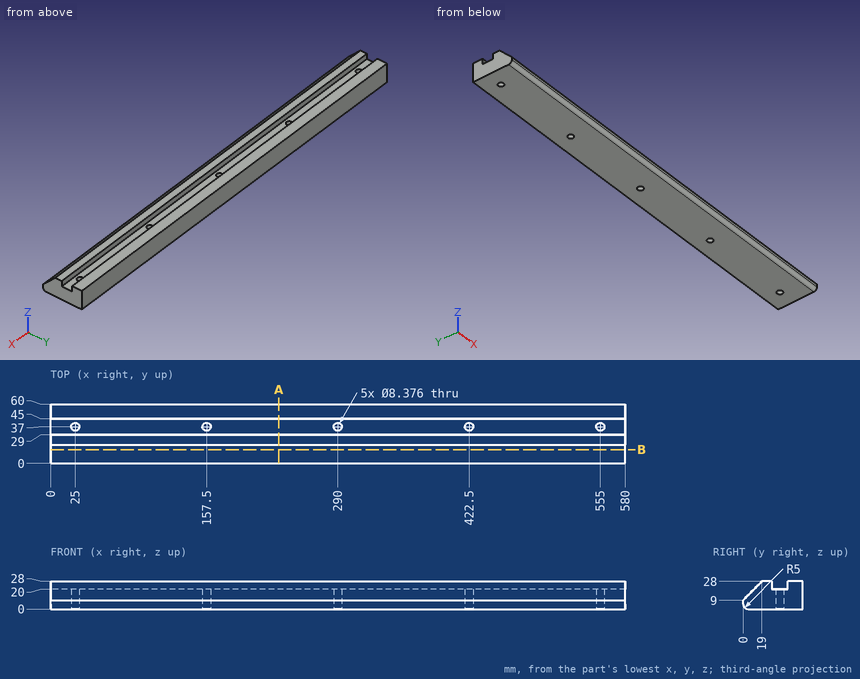
Input: dimensioned drawing with shaded views. Units: mm. Origin: part minimum x, y, z. Give positions to 0.01 mm unless a question says otherwise; leave off trailing zeros. Write each loop counter-clockwise with the first axis right and the second up, starting at its lowest first coordinate (ties: lowest second). Pieces come first, ordered by that corner, then holes.
1. Section query B-B (y = 14). Return the cut outline in (x, z).
2. First-contact query: pin 1 (9 mm diameter, centred on x = 200.5, z = 22, fed in from -Y); pin 2 (3 mm diameter, centred on x = 138.5, y = 35.5, fed in from +Z); pin 3 (10 mm diameter, centred on x = 162.5, z = 19, fed in from -Y). Flat tips, straight axial feed; report the tip coordinate or a pass-through.
3. Material intervals for line 1 along X through (y, z) = (37, 14.25); line 2 along X through (y, z) = (36, 17.5); line 3 along Y through (x, z) = (422.5, 8.25), sorted ascending.
4. Section query A-A (x = 230.5). Return the cut outline in (y, z), then the cut area to 3 significant figures.
Output values:
1. outline: (0, 0) - (580, 0) - (580, 23) - (0, 23) - close
2. pin 1: stops at y = 8.5
2. pin 2: stops at z = 20
2. pin 3: stops at y = 5
3. line 1: x = 0 to 20.81, 29.19 to 153.31, 161.69 to 285.81, 294.19 to 418.31, 426.69 to 550.81, 559.19 to 580
3. line 2: x = 0 to 20.93, 29.07 to 153.43, 161.57 to 285.93, 294.07 to 418.43, 426.57 to 550.93, 559.07 to 580
3. line 3: y = 0 to 32.81, 41.19 to 60
4. outline: (0, 5) arc R5 ccw to (5, 0) - (60, 0) - (60, 28) - (45, 28) - (45, 20) - (29, 20) - (29, 28) - (19, 28) - (0, 9) - close
4. area: 1,370 mm2
